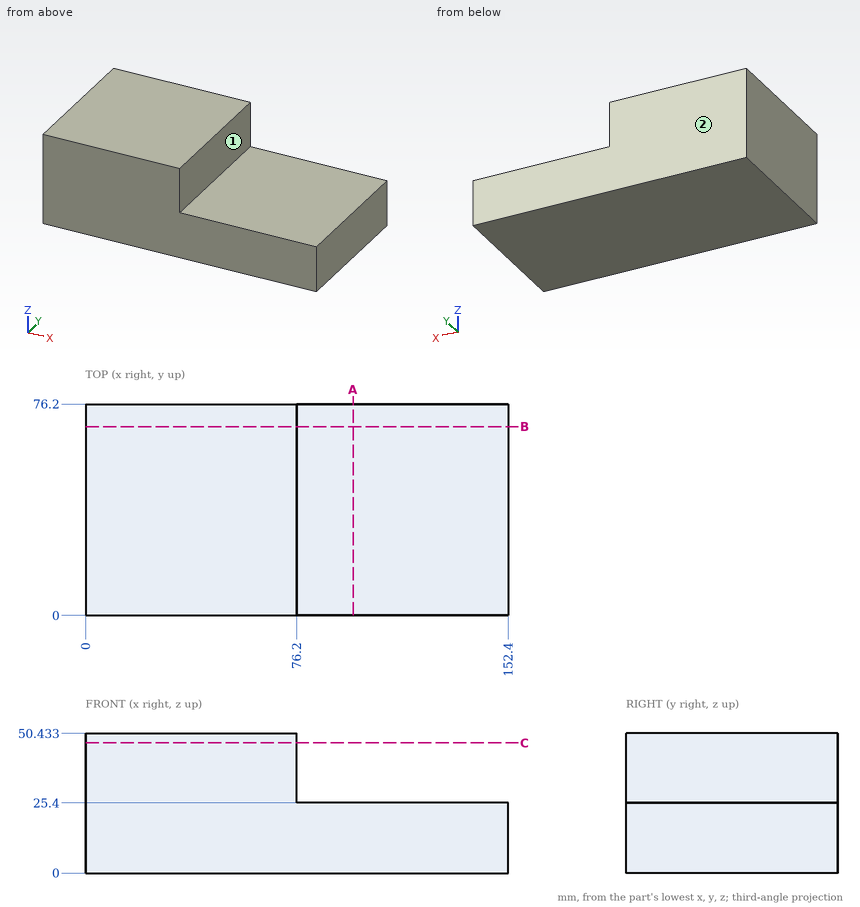
Geometry check sheet. Reference: drawing and pictorial views, mm from the part's lowest x, y, z. A direction names the side the tool comes from. Give positions to 0.01 mm unless a question says otherwise; leave off trailing zeros. Order: outer loops, then holes, each group sorted by start corner. A loop starts at its lowest first (then second) coordinate and runs counter-clockwise, first axis right, second up. Notation, with made-up numbers: M 87.25,-15 L 144.25,-15 A22 cw 144.25,14 Z; hole C -8,-5.5 d10. An arc over 180 degrees is marked long. Answer in a Markdown table with one row per item. Add a question column.
Q1. Sectioned sample at A-A, the plane x = 96.5. Record the boundary of the cut face in (y, z).
Q2. Thickness scan on L1, parallel to X at y = 67, z = 29.5; L2, parallel to Z at x = 97, y = 73. Record the ranges inside material, lowest first.
Q3. Sectioned sample at C-C, the plane z = 47. Record the boundary of the cut face in (x, y).
Q4. Access from +Z, -Z, +X, -X, +Y, -Y to the whole of each face (thin tool, end or side, straight path). Record for the marked faces 1 and 2.
Q5. Gauge pin test, flat ends, axial feed: pin 1 Ø10 at (x, y) = (129, 42) entering from +Z; pin 2 Ø20 at (y, z) = (31.5, 43) entering from +X. Record the tip position at first contact, or that the pin passes through.
Q6. Sectioned sample at B-B, the plane y = 68. Record the boundary of the cut face in (x, z), and give its area (3 significant figures).
Verdict:
| question | item | result |
|---|---|---|
| 1 | outline | M 0,0 L 76.2,0 L 76.2,25.4 L 0,25.4 Z |
| 2 | L1 | 0 to 76.2 |
| 2 | L2 | 0 to 25.4 |
| 3 | outline | M 0,0 L 76.2,0 L 76.2,76.2 L 0,76.2 Z |
| 4 | face 1 | +Z, +X, +Y, -Y |
| 4 | face 2 | +Z, -Z, +X, -X, +Y |
| 5 | pin 1 | z = 25.4 |
| 5 | pin 2 | x = 76.2 |
| 6 | outline | M 0,0 L 152.4,0 L 152.4,25.4 L 76.2,25.4 L 76.2,50.43 L 0,50.43 Z |
| 6 | area | 5,780 mm² |
